CAD build for the part. Positions are in the model's coordinates, mm. Face numbers are marked on the shaded views. A direction names the side the tool comes from. Give positions to 0.01 mm unless a question says otherwise; leave off trailing zeros. Write each loop counter-clockwise with the first axis right and the second up, starting at its lowest first coordinate (ties: lowest second). Pieces come first, ordered by that corner, then holes. Notation, with made-up numbers: (-40, 83) - (-35, 83) arc R16 cw to (-35, 109) - close; hole circle Ø1 at (-3, 26.25). An arc over 180 degrees is marked (long way). Answer as a JSON object with one key per item and string values.
from build123d import *

# Parameters (mm, degrees)
BOSS_EXTRUDE1_DEPTH = 10
BOSS_EXTRUDE2_DEPTH = 6.5
SKETCH4_R           = 3
SKETCH4_R_2         = 3.0000000000000084
CUT_EXTRUDE2_DEPTH  = 10
BOSS_EXTRUDE3_DEPTH = 60
BOSS_EXTRUDE5_DEPTH = 4
CUT_EXTRUDE3_DEPTH  = 186.5693940282179
FILLET2_R           = 3
CUT_EXTRUDE4_DEPTH  = 187.81541692269406
FILLET3_R           = 1.25
SKETCH9_OUTSIDE_W   = 170.05200000000002
SKETCH9_OUTSIDE_H   = 160.05200000000002
SKETCH9_OUTSIDE_W_2 = 23.614386219061117
SKETCH9_OUTSIDE_H_2 = 74.99999999999999
CUT_EXTRUDE6_DEPTH  = 10
CUT_EXTRUDE7_DEPTH  = 60


with BuildPart() as part:
    # Sketch2 → Boss-Extrude1 (new body)
    with BuildSketch(Plane.XY):
        Polygon((0, 0), (130, 0), (130, 14), (75, 69), (75, 120.00000000000001), (-2.45e-15, 120), align=None)
    extrude(amount=-BOSS_EXTRUDE1_DEPTH)

    # Sketch3 → Boss-Extrude2 (add)
    with BuildSketch(Plane.XY):
        Polygon((-2.45e-15, 120), (75, 120), (75, 116.99999999999999), (-2.08e-15, 117), align=None)
        Polygon((-2.45e-15, 80.99999999999999), (75, 80.99999999999999), (75, 77.99999999999999), (-2.08e-15, 77.99999999999999), align=None)
    extrude(amount=BOSS_EXTRUDE2_DEPTH)

    # Sketch4 → Cut-Extrude2 (cut)
    with BuildSketch(Plane.XY):
        with Locations((10.000000000000002, 98.99999999999999)):
            Circle(SKETCH4_R)
        with Locations((65, 98.99999999999997)):
            Circle(SKETCH4_R_2)
    extrude(amount=-CUT_EXTRUDE2_DEPTH, mode=Mode.SUBTRACT)

    # Sketch5 → Boss-Extrude3 (add)
    with BuildSketch(Plane.XY):
        Polygon((130, 14), (104.00000000000001, 13.999999999999995), (104.00000000000001, 4.78e-15), (130, 0), align=None)
        Polygon((7.999999999999998, 0), (34, 0), (34, 13.999999999999995), (7.999999999999993, 14), align=None)
    extrude(amount=BOSS_EXTRUDE3_DEPTH)

    # Sketch7 → Boss-Extrude5 (add)
    with BuildSketch(Plane.XY):
        with BuildLine():
            Line((52.99999999999999, 13.00000000000001), (53, 60.00000000000001))
            ThreePointArc((53, 60.00000000000001), (60, 67), (67, 60.00000000000001))
            Line((67, 60.00000000000001), (67, 13.00000000000001))
            ThreePointArc((67, 13.00000000000001), (60, 6.0000000000000036), (52.99999999999999, 13.00000000000001))
        make_face()
    extrude(amount=BOSS_EXTRUDE5_DEPTH)

    # Sketch8 → Cut-Extrude3 (cut, through all)
    with BuildSketch(Plane.XY.offset(4)):
        with BuildLine():
            Line((62.2, 13.00000000000001), (62.2, 60.00000000000001))
            ThreePointArc((62.2, 60.00000000000001), (60, 62.20000000000001), (57.8, 60.00000000000001))
            Line((57.8, 60.00000000000001), (57.79999999999999, 13.00000000000001))
            ThreePointArc((57.79999999999999, 13.00000000000001), (60, 10.8), (62.2, 13.00000000000001))
        make_face()
    extrude(amount=-CUT_EXTRUDE3_DEPTH, mode=Mode.SUBTRACT)

    # Fillet2
    fillet2_edges = [part.edges().sort_by_distance(p)[0] for p in [
        (75, 120, -1.75),
        (-2.45e-15, 120, -1.75),
        (37.5, 77.99999999999999, 0),
        (75, 69, -5),
    ]]
    fillet(fillet2_edges, radius=FILLET2_R)

    # Sketch6 → Cut-Extrude4 (cut, through all)
    with BuildSketch(Plane.XY):
        Polygon((-2.08e-15, 13.000000000000002), (5.999999999999998, 6.999999999999992), (5.999999999999998, 24.999999999999993), (-2.82e-15, 19), align=None)
        Polygon((5.999999999999998, 47), (-4.68e-15, 52.99999999999999), (-4.68e-15, 59), (5.999999999999998, 65), align=None)
    extrude(amount=-CUT_EXTRUDE4_DEPTH, mode=Mode.SUBTRACT)

    # Fillet3
    fillet3_edges = [part.edges().sort_by_distance(p)[0] for p in [
        (-2.08e-15, 13.000000000000002, -5),
        (-2.82e-15, 19, -5),
        (5.999999999999998, 24.999999999999993, -5),
        (5.999999999999998, 6.999999999999992, -5),
        (5.999999999999998, 65, -5),
        (5.999999999999998, 47, -5),
        (-4.68e-15, 52.99999999999999, -5),
        (-4.68e-15, 59, -5),
    ]]
    fillet(fillet3_edges, radius=FILLET3_R)

    # Sketch9 outside → Cut-Extrude6 (cut)
    with BuildSketch(Plane.XY):
        with Locations((65, 60.00000000000001)):
            Rectangle(SKETCH9_OUTSIDE_W, SKETCH9_OUTSIDE_H)
        with Locations((11.807193109530559, 37.49999999999999)):
            Rectangle(SKETCH9_OUTSIDE_W_2, SKETCH9_OUTSIDE_H_2, mode=Mode.SUBTRACT)
    extrude(amount=-CUT_EXTRUDE6_DEPTH, mode=Mode.SUBTRACT)


with BuildPart() as body_2:
    # of the pieces the cut leaves, the one that is kept (cut_extrude6_keep)
    add(part.part.solids().sort_by_distance((0, 62.017766953, 0))[0])

    # Sketch10 → Cut-Extrude7 (cut)
    with BuildSketch(Plane.XY.offset(60)):
        Polygon((7.999999999999993, 14), (7.999999999999998, 0), (34, 0), (34, 13.999999999999995), align=None)
    extrude(amount=-CUT_EXTRUDE7_DEPTH, mode=Mode.SUBTRACT)


solid = body_2.part
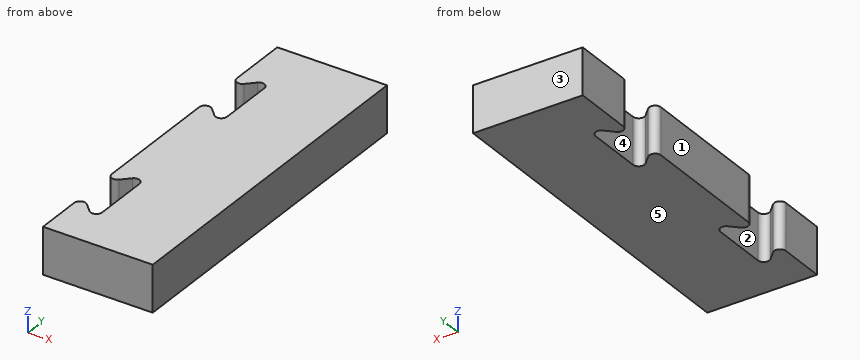
(1) Saw through at B-B, the plane x = 5. Give the cut face in (y, z).
Answer key:
{"outline": "(0, -10) - (8.79, -10) - (8.79, 0) - (0, 0) - close; (23.21, -10) - (48.79, -10) - (48.79, 0) - (23.21, 0) - close; (63.21, -10) - (75, -10) - (75, 0) - (63.21, 0) - close"}
(2) Saw through at C-C, the plane y = 57.5. Give the cut face in (x, z).
Answer key:
{"outline": "(6, -10) - (23.61, -10) - (23.61, 0) - (6, 0) - close"}
(3) Saw through at A-A, the plane z = -4.5. Give the cut face in (x, y), and give its area (3 significant figures).
Answer key:
{"outline": "(0, 0) - (23.61, 0) - (23.61, 75) - (0, 75) - (0, 62.02) arc R1.25 ccw to (2.13, 61.13) - (3.87, 62.87) arc R1.25 cw to (6, 61.98) - (6, 50.02) arc R1.25 cw to (3.87, 49.13) - (2.13, 50.87) arc R1.25 ccw to (0, 49.98) - (0, 22.02) arc R1.25 ccw to (2.13, 21.13) - (3.87, 22.87) arc R1.25 cw to (6, 21.98) - (6, 10.02) arc R1.25 cw to (3.87, 9.13) - (2.13, 10.87) arc R1.25 ccw to (0, 9.98) - close", "area": "1,630 mm²"}
(4) 3-axis set-ups, long thin cutter, end or side, ignore diameter. For the marked faces 4 and 5: which of +Z, -Z, +X, -X, +Y, -Y reach the whole face in a straight line?
Answer key:
{"face 4": "+Z, -Z", "face 5": "-Z, +X, -X, +Y, -Y"}
(5) Probe L1, parallel to Y at x = 5.5, z = -4; L2, parallel to Y at x = 1.75, z = -3; L3, parallel to X at y = 17, z = -7. List the from-to ranges inside material, lowest first. Write a range as [from, to].
Answer key:
{"L1": "y = [0, 9.02], [22.98, 49.02], [62.98, 75]", "L2": "y = [0, 11.13], [20.87, 51.13], [60.87, 75]", "L3": "x = [6, 23.61]"}
(6) Pull direction Y, two halves, no side cores. Call the marked faces 1, 2 and 3: pulls with the +Y half, pulls with the -Y half, needs draft (parallel to the pull), parting line crosses it, or undercut.
Answer key:
{"face 1": "needs draft", "face 2": "undercut", "face 3": "pulls with the +Y half"}
(7) Flat gauge pin, fed straight in: P1, Ø5, axis at y = 15.5, z = -4.5, coming from the -X side. Where does the tip first touch, or does it go through?
Answer key:
{"P1": "stops at x = 6"}
